Model file for the job. Use its own axes, mm. A direction names the side the tool comes from. Round coordinates to 2 decimals unless told otherwise and drop trailing zeros. Loops run counter-clockwise (first coordinate to the right, second up) from the corner with the lowest first, then second, coordinate; pieces in that order, holes last. Notation, with made-up numbers: (82.5, -4) -> (101.5, -4) arc R27 cw to (101.5, 28) -> close; hole circle Ø1 at (-14.5, 25). An arc over 180 degrees is marked (long way). Use a Markdown table: item, result.
from build123d import *

# Parameters (mm, degrees)
F0_W     = 140.7
F0_H     = 280
F1_DEPTH = 25
F2_R     = 174.3309751569
F3_DEPTH = 25


with BuildPart() as f1:
    # F0 (on Top) → F1 (new body)
    with BuildSketch(Plane.XY):
        with Locations((0.5157602191, -46.0708594322)):
            Rectangle(F0_W, F0_H)
    extrude(amount=F1_DEPTH)

    # F2 (on Top) → F3 (join)
    with BuildSketch(Plane.XY):
        with Locations((0, -127.1062195301)):
            Circle(F2_R)
        with BuildLine():
            ThreePointArc((135.9251850135, -117.1062195301), (136.2006688085, -122.1028469617), (136.2925380237, -127.1062195301))
            ThreePointArc((136.2925380237, -127.1062195301), (136.2006688085, -132.1095920985), (135.9251850135, -137.1062195301))
            ThreePointArc((135.9251850135, -137.1062195301), (128.2461669599, -173.2427189751), (111.1444855362, -205.9894196163))
            ThreePointArc((111.1444855362, -205.9894196163), (105.0571290732, -213.9316510109), (98.4034458961, -221.4058364791))
            ThreePointArc((98.4034458961, -221.4058364791), (58.0603027008, -250.4133854664), (10, -263.0314045436))
            ThreePointArc((10, -263.0314045436), (0, -263.3987575538), (-10, -263.0314045436))
            ThreePointArc((-10, -263.0314045436), (-57.3758238008, -250.7333636536), (-97.3518624436, -222.4910757689))
            ThreePointArc((-97.3518624436, -222.4910757689), (-104.0880057129, -215.0911215739), (-110.2630464775, -207.2168711467))
            ThreePointArc((-110.2630464775, -207.2168711467), (-127.9884260341, -173.9529773929), (-135.9251850135, -137.1062195301))
            ThreePointArc((-135.9251850135, -137.1062195301), (-136.2925380237, -127.1062195301), (-135.9251850135, -117.1062195301))
            ThreePointArc((-135.9251850135, -117.1062195301), (0, 9.1863184936), (135.9251850135, -117.1062195301))
        make_face(mode=Mode.SUBTRACT)
        with BuildLine():
            ThreePointArc((111.4590298101, -127.1062195301), (111.3465976726, -122.1011707841), (111.0095280875, -117.1062195301))
            ThreePointArc((111.0095280875, -117.1062195301), (0, -15.64718972), (-111.0095280875, -117.1062195301))
            ThreePointArc((-111.0095280875, -117.1062195301), (-111.4590298101, -127.1062195301), (-111.0095280875, -137.1062195301))
            ThreePointArc((-111.0095280875, -137.1062195301), (-104.667988428, -165.4171517121), (-91.2347043683, -191.1323395519))
            ThreePointArc((-91.2347043683, -191.1323395519), (-85.1224014158, -199.0596218362), (-78.3235203344, -206.4065441741))
            ThreePointArc((-78.3235203344, -206.4065441741), (-46.9215244512, -228.2075838601), (-10, -238.1157476176))
            ThreePointArc((-10, -238.1157476176), (0, -238.5652493402), (10, -238.1157476176))
            ThreePointArc((10, -238.1157476176), (47.4812862344, -227.9459080646), (79.197938217, -205.5332678514))
            ThreePointArc((79.197938217, -205.5332678514), (85.9149433339, -198.1114153833), (91.9389778571, -190.1168509886))
            ThreePointArc((91.9389778571, -190.1168509886), (104.8787670513, -164.8363076298), (111.0095280875, -137.1062195301))
            ThreePointArc((111.0095280875, -137.1062195301), (111.3465976726, -132.1112682761), (111.4590298101, -127.1062195301))
        make_face()
        with BuildLine():
            ThreePointArc((-10, -263.0314045436), (0, -263.3987575538), (10, -263.0314045436))
            Line((10, -263.0314045436), (10, -238.1157476176))
            ThreePointArc((10, -238.1157476176), (0, -238.5652493402), (-10, -238.1157476176))
            Line((-10, -238.1157476176), (-10, -263.0314045436))
        make_face()
        with BuildLine():
            Line((-111.0095280875, -117.1062195301), (-135.9251850135, -117.1062195301))
            ThreePointArc((-135.9251850135, -117.1062195301), (-136.2925380237, -127.1062195301), (-135.9251850135, -137.1062195301))
            Line((-135.9251850135, -137.1062195301), (-111.0095280875, -137.1062195301))
            ThreePointArc((-111.0095280875, -137.1062195301), (-111.4590298101, -127.1062195301), (-111.0095280875, -117.1062195301))
        make_face()
        with BuildLine():
            Line((-91.2347043683, -191.1323395519), (-110.2630464775, -207.2168711467))
            ThreePointArc((-110.2630464775, -207.2168711467), (-104.0880057129, -215.0911215739), (-97.3518624436, -222.4910757689))
            Line((-97.3518624436, -222.4910757689), (-78.3235203344, -206.4065441741))
            ThreePointArc((-78.3235203344, -206.4065441741), (-85.1224014158, -199.0596218362), (-91.2347043683, -191.1323395519))
        make_face()
        with BuildLine():
            ThreePointArc((98.4034458961, -221.4058364791), (105.0571290732, -213.9316510109), (111.1444855362, -205.9894196163))
            Line((111.1444855362, -205.9894196163), (91.9389778571, -190.1168509886))
            ThreePointArc((91.9389778571, -190.1168509886), (85.9149433339, -198.1114153833), (79.197938217, -205.5332678514))
            Line((79.197938217, -205.5332678514), (98.4034458961, -221.4058364791))
        make_face()
        with BuildLine():
            ThreePointArc((135.9251850135, -137.1062195301), (136.2006688085, -132.1095920985), (136.2925380237, -127.1062195301))
            ThreePointArc((136.2925380237, -127.1062195301), (136.2006688085, -122.1028469617), (135.9251850135, -117.1062195301))
            Line((135.9251850135, -117.1062195301), (111.0095280875, -117.1062195301))
            ThreePointArc((111.0095280875, -117.1062195301), (111.3465976726, -122.1011707841), (111.4590298101, -127.1062195301))
            ThreePointArc((111.4590298101, -127.1062195301), (111.3465976726, -132.1112682761), (111.0095280875, -137.1062195301))
            Line((111.0095280875, -137.1062195301), (135.9251850135, -137.1062195301))
        make_face()
    extrude(amount=F3_DEPTH)


solid = f1.part
Q1. Pull direction X, two halves, no side cores. Call faces 4 (the face through (70.866, 63, 12)), 5 (the face through (-123, -117.106, 12)), 6 (the face through (-7.215, -301.288, 12.325)): released by +X, released by -X, zero draft, split by the parting line, or undercut.
Results list:
| item | result |
|---|---|
| face 4 | released by +X |
| face 5 | undercut |
| face 6 | split by the parting line |
Q2. Drill centre lines: L1, parallel to Y at x = 119.5, z = 22; L2, parallel to X at y = -164, z = 6.5; L3, parallel to Y at x = 86.5, z = 18.75. Where is each one in solid material? Low to high. Write a range as from..to.
Results list:
| item | result |
|---|---|
| L1 | y = -254.04..-192.65, -137.11..-117.11, -61.57..-0.18 |
| L2 | x = -170.38..-131.2, -105.18..105.18, 131.2..170.38 |
| L3 | y = -278.46..-232.43, -211.57..-56.81, -21.78..24.25 |
Q3. Flat gauge pins, fed straight in: pin 1 (7.5 mm diameter, centred on y = -250, z = 17, fed in from -X); pin 2 (7.5 mm diameter, centred on x = -127, z = 8, fed in from +Y) (3 decimals); pin 3 (1 mm diameter, centred on y = 49, z = 19.5, fed in from +X); pin 4 (10 mm diameter, centred on x = -60, y = -255, fed in from -Z). Where does each tip first touch, or does it go through?
Results list:
| item | result |
|---|---|
| pin 1 | stops at x = -127.26 |
| pin 2 | stops at y = -3.815 |
| pin 3 | stops at x = 70.87 |
| pin 4 | stops at z = 0 |
Q4. Band-saw the part on B-B, the plane z = 17.75. Give the cut face in (x, y).
Results list:
| item | result |
|---|---|
| outline | (-69.83, 32.63) arc R174.33 ccw (long way) to (70.87, 32.17) -> (70.87, 93.93) -> (-69.83, 93.93) -> close; hole (-135.93, -137.11) arc R136.29 ccw to (-110.26, -207.22) -> (-91.23, -191.13) arc R111.46 cw to (-111.01, -137.11) -> close; hole (-135.93, -117.11) -> (-111.01, -117.11) arc R111.46 cw to (-69.83, -40.24) -> (-69.83, -10.06) arc R136.29 ccw to start; hole (-97.35, -222.49) arc R136.29 ccw to (-10, -263.03) -> (-10, -238.12) arc R111.46 cw to (-78.32, -206.41) -> close; hole (10, -263.03) arc R136.29 ccw to (98.4, -221.41) -> (79.2, -205.53) arc R111.46 cw to (10, -238.12) -> close; hole (70.87, -41.08) arc R111.46 cw to (111.01, -117.11) -> (135.93, -117.11) arc R136.29 ccw to (70.87, -10.69) -> close; hole (91.94, -190.12) -> (111.14, -205.99) arc R136.29 ccw to (135.93, -137.11) -> (111.01, -137.11) arc R111.46 cw to start |
Q5. Band-saw the part on C-C, the plane x = 53.5. Give the cut face in (y, z) (3 decimals).
Results list:
| item | result |
|---|---|
| outline | (-293.025, 0) -> (-252.459, 0) -> (-252.459, 25) -> (-293.025, 25) -> close; (-224.886, 0) -> (93.929, 0) -> (93.929, 25) -> (-224.886, 25) -> close |
Q6. Tool access for faces 1 (the face through (-69.834, 63, 12)), 2 (the face through (98.85, -75.61, 12.32)), 3 (the face through (0, 93.929, 12)): list every direction of +Z, -Z, +X, -X, +Y, -Y with a clear straight run to the whole face (end or side of a thin tool).
Results list:
| item | result |
|---|---|
| face 1 | +Z, -Z, -X, +Y |
| face 2 | +Z, -Z |
| face 3 | +Z, -Z, +X, -X, +Y |
Q7. Band-saw the part on A-A, the plane y = -155.5. Give the cut face in (x, z), plus the area to 3 significant figures.
Results list:
| item | result |
|---|---|
| outline | (-172, 0) -> (-133.3, 0) -> (-133.3, 25) -> (-172, 25) -> close; (-107.78, 0) -> (107.78, 0) -> (107.78, 25) -> (-107.78, 25) -> close; (133.3, 0) -> (172, 0) -> (172, 25) -> (133.3, 25) -> close |
| area | 7,320 mm² |
Q8. Band-saw the part on D-D, the plane x = 103. Give the cut face in (y, z).
Results list:
| item | result |
|---|---|
| outline | (-267.76, 0) -> (-199.26, 0) -> (-199.26, 25) -> (-267.76, 25) -> close; (-169.7, 0) -> (-84.51, 0) -> (-84.51, 25) -> (-169.7, 25) -> close; (-37.85, 0) -> (13.54, 0) -> (13.54, 25) -> (-37.85, 25) -> close |
